The listing builds one solid part. Answer for the finished solid, in the listing's coordinates (mm). Face numbers are marked on the shaded views. A direction names the side the tool comes from. Give positions to 0.01 mm unless a question says otherwise; leave off trailing zeros. Loops run counter-clockwise (first coordinate to the right, second up) from the corner with the lowest first, then second, coordinate; pieces in that order, holes last. Notation, with made-up numbers: M -11,-3.5 L 15,-3.5 A24 ccw 15,17.5 Z; hole C 5.25,24 d7. An arc over 180 degrees is marked long. Return JSON: item names as keys, results as strings.
from build123d import *

# Parameters (mm, degrees)
EXTRUDE_1_DEPTH     = 25
CUT_EXTRUDE_3_DEPTH = 1
CUT_EXTRUDE_START   = -1
CUT_EXTRUDE_4_DEPTH = 1
CHAMFER_1_SIZE      = 1
EXTRUDE_2_DEPTH     = 3.5
EXTRUDE_START       = 3.5
EXTRUDE_3_DEPTH     = 3.5
FILLET_1_R          = 0.5
SKETCH_6_R          = 4
CUT_EXTRUDE_5_DEPTH = 63.165102751


with BuildPart() as part:
    # ｽｹｯﾁ1 → ﾎﾞｽ - 押し出し1 (new body)
    with BuildSketch(Plane(origin=(0, 0, 0), x_dir=(1, 0, 0), z_dir=(0, 1, 0))):
        with BuildLine():
            ThreePointArc((35.980947353, 13.697497128), (22.958239241, 30.905812576), (2.722143787, 38.403644791))
            ThreePointArc((2.722143787, 38.403644791), (-28.169598292, -26.243546485), (38.5, 0))
            ThreePointArc((38.5, 0), (37.865000153, 6.963602764), (35.980947353, 13.697497128))
        make_face()
    extrude(amount=EXTRUDE_1_DEPTH)

    # ｽｹｯﾁ2 → ｶｯﾄ - 押し出し3 (cut)
    with BuildSketch(Plane(origin=(0, 25, 0), x_dir=(1, 0, 0), z_dir=(0, 1, 0))):
        with BuildLine():
            ThreePointArc((34.036718994, 11.726114452), (21.467444485, 28.898941629), (1.396281143, 35.972912017))
            ThreePointArc((1.396281143, 35.972912017), (-25.94480797, -24.957302327), (36, 0))
            ThreePointArc((36, 0), (35.505787442, 5.944666358), (34.036718994, 11.726114452))
        make_face()
    extrude(amount=-CUT_EXTRUDE_3_DEPTH, mode=Mode.SUBTRACT)

    # ｽｹｯﾁ3 → ｶｯﾄ - 押し出し4 (cut)
    with BuildSketch(Plane.XZ.offset(CUT_EXTRUDE_START)):
        with BuildLine():
            ThreePointArc((34.036718994, 11.726114452), (21.467444485, 28.898941629), (1.396281143, 35.972912017))
            ThreePointArc((1.396281143, 35.972912017), (-25.94480797, -24.957302327), (36, 0))
            ThreePointArc((36, 0), (35.505787442, 5.944666358), (34.036718994, 11.726114452))
        make_face()
    extrude(amount=CUT_EXTRUDE_4_DEPTH, mode=Mode.SUBTRACT)

    # 面取り1
    chamfer_1_edges = [part.edges().sort_by_distance(p)[0] for p in [
        (-36, 1, 0),
        (-36, 24, 0),
    ]]
    chamfer(chamfer_1_edges, length=CHAMFER_1_SIZE - 0.0001)  # a hair under: the kernel refuses the full size

    # ｽｹｯﾁ4 → ﾎﾞｽ - 押し出し2 (add)
    with BuildSketch(Plane.XZ.offset(-1)):
        with BuildLine():
            ThreePointArc((21.5, 0), (11.339952646, 18.266238638), (-9.537718509, 19.268677319))
            ThreePointArc((-9.537718509, 19.268677319), (-12.820834901, -17.25909014), (21.202158445, -3.566297417))
            ThreePointArc((21.202158445, -3.566297417), (21.425410224, -1.789356508), (21.5, 0))
        make_face()
    extrude(amount=EXTRUDE_2_DEPTH)

    # ｽｹｯﾁ5 → ﾎﾞｽ - 押し出し3 (add)
    with BuildSketch(Plane(origin=(0, 24, 0), x_dir=(1, 0, 0), z_dir=(0, 1, 0)).offset(EXTRUDE_START)):
        with BuildLine():
            ThreePointArc((21.5, 0), (11.339952646, 18.266238638), (-9.537718509, 19.268677319))
            ThreePointArc((-9.537718509, 19.268677319), (-12.820834901, -17.25909014), (21.202158445, -3.566297417))
            ThreePointArc((21.202158445, -3.566297417), (21.425410224, -1.789356508), (21.5, 0))
        make_face()
    extrude(amount=-EXTRUDE_3_DEPTH)

    # ﾌｨﾚｯﾄ1
    fillet_1_edges = [part.edges().sort_by_distance(p)[0] for p in [
        (-21.202158445, -2.5, 3.566297417),
        (-21.202158445, 27.5, -3.566297417),
    ]]
    fillet(fillet_1_edges, radius=FILLET_1_R)

    # ｽｹｯﾁ6 → ｶｯﾄ - 押し出し5 (cut, through all)
    with BuildSketch(Plane.XZ.offset(2.5)):
        with Locations(Location((0, 0, 0), (0, 0, 270))):
            Circle(SKETCH_6_R)
    extrude(amount=-CUT_EXTRUDE_5_DEPTH, mode=Mode.SUBTRACT)


solid = part.part
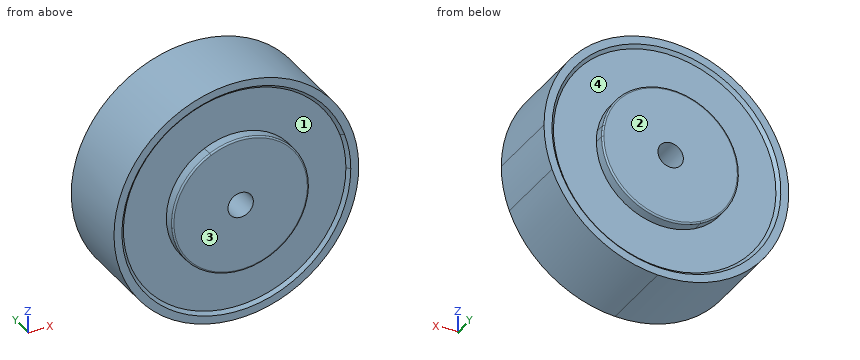
(1) Straight lines are drawn through the part: line 1 along Y through (x, z) = (33, -18); line 2 along Y through (x, z) = (-22, 12); line 3 along X through (y, z) = (24.25, -26). For each, find the intervals that lie inside material, in ascending order.
Values follow:
{"line 1": "0 to 25", "line 2": "1 to 24", "line 3": "-28.39 to -23.8, 23.8 to 28.39"}
(2) A tool of negligible diameter and unlimited length cuts with its end or side. For the marked faces 3 and 4, from which of +Z, -Z, +X, -X, +Y, -Y can it reach the whole face along a straight path? Write none if from no direction.
Values follow:
{"face 3": "+Z, -Z, +X, -X, -Y", "face 4": "+Y"}
(3) Given pin 1 (4 mm diameter, centred on y = 13, z = 3, fed in from -X); pin 2 (1.5 mm diameter, centred on x = -21, z = -24, fed in from +Y); pin 3 (6 mm diameter, centred on y = 18, z = -25.5, fed in from -X); pin 4 (6.5 mm diameter, centred on x = 0, z = 0, fed in from +Y), each flat-ended and moving along its own axis, determine where each tip first touches the part or whether it passes through.
Values follow:
{"pin 1": "x = -38.49", "pin 2": "y = 24", "pin 3": "x = -31.24", "pin 4": "through"}
(4) The part is cut by section A-A (y = 5). Determine the outline of the cut face in (x, z), and give its area (3 significant figures).
Values follow:
{"outline": "C 0,0 d77; hole C 0,0 d8", "area": "4,610 mm²"}
(5) Determine the mould class of the marked faces 1 and 2 for opening direction Z: released by +Z, released by -Z, zero draft, split by the parting line, or undercut.
Values follow:
{"face 1": "undercut", "face 2": "zero draft"}
